Autodesk Inventor part; units mm, degrees
ref_plane "Work Plane1" through (0, 0, 12.7) normal (0, 0, 1) x (1, 0, 0)
ref_plane "Work Plane2" through (0, 0, -12.7) normal (0, 0, -1) x (-1, 0, 0)
ref_plane "YZ Plane" through (0, 0, 0) normal (1, 0, 0) x (0, 1, 0)
sketch "Sketch1" plane through (0, 0, 0) normal (0, 0, 1) x (1, 0, 0)
  line L0 (0, 0) -> (0, 12.7)
  line L1 (0, 12.7) -> (-25.952, 3.0759)
  line L2 (0, 0) -> (-25.4, 0)
  arc A0 (-25.952, 3.0759) -> (-25.4, 0) centre (-25.4, 1.5875) ccw
  dimension "d0" = 25.4
  dimension "d1" = 3.175
  dimension "d2" = 12.7
extrude "Extrusion1" add sketch "Sketch1" along normal mid plane 5.08
ref_plane "Work Plane1" through (0, 0, 12.7) normal (0, 0, 1) x (1, 0, 0)
sketch "Sketch2" plane through (0, 0, 12.7) normal (0, 0, 1) x (1, 0, 0)
  arc A0 (-32.2031, 3.109) -> (-31.75, 0) centre (-31.75, 1.5875) ccw
  line L0 (0, 0) -> (-31.75, 0)
  line L1 (0, 0) -> (0, 12.7)
  line L2 (0, 12.7) -> (-32.2031, 3.109)
  line L3 (0, 12.7) -> (-25.952, 3.0759) construction
  dimension "d6" = 3.175
  dimension "d7" = 31.75
ref_plane "Work Plane2" through (0, 0, -12.7) normal (0, 0, -1) x (-1, 0, 0)
sketch "Sketch3" plane through (0, 0, -12.7) normal (0, 0, -1) x (-1, 0, 0)
  line L0 (0, 12.7) -> (32.2031, 3.109)
  arc A0 (31.75, 0) -> (32.2031, 3.109) centre (31.75, 1.5875) ccw
  line L1 (0, 0) -> (31.75, 0)
  line L2 (0, 0) -> (0, 12.7)
loft "Loft1" add profiles "Sketch2" section 1 edges at (0, 6.35, 2.54) (-12.976, 7.888, 2.54) (-26.9625, 1.3071, 2.54) (-12.7, 0, 2.54)
loft "Loft2" add profiles "Sketch3" section 1 edges at (0, 6.35, -2.54) (-12.7, 0, -2.54) (-26.9625, 1.3071, -2.54) (-12.976, 7.888, -2.54)
sketch "Sketch4" plane through (0, 0, 12.7) normal (1, 0, 0) x (0, 0, -1)
  line L0 (15.24, 12.7) -> (10.16, 12.7) construction
  line L1 (10.16, 12.7) -> (0, 12.7) construction
  line L2 (0, 12.7) -> (0, 0) construction
  line L3 (0, 0) -> (25.4, 0) construction
  line L4 (25.4, 0) -> (25.4, 12.7) construction
  line L5 (15.24, 12.7) -> (25.4, 12.7) construction
  line L6 (0, 12.7) -> (12.7, 0) construction
  line L7 (12.7, 0) -> (25.4, 12.7) construction
  circle A0 centre (6.35, 6.35) radius 1.5875
  circle A1 centre (19.05, 6.35) radius 1.5875
  dimension "d17" = 3.175
  dimension "d18" = 3.175
extrude "Extrusion2" add sketch "Sketch4" along normal blind 6.35
properties part number "Bottom Pivot Mk1"
For this review, take the finished solid that the model builds, in its own axes (mm). A direction names the side the tool comes from. Round coordinates to 2 decimals unless told otherwise and drop trailing zeros. Loops run counter-clockwise (first coordinate to the right, second up) from the corner with the lowest first, then second, coordinate; pieces in that order, holes last.
Q1. Mouldability with a two-part tool opening along Z and no side actions: class faces 1 (the face through (-12, 4, 12.7)), 2 (the face through (-12, 0, 0)), 3 (the face through (3.131, 7.316, -5.09)) as +Z half, -Z half, draft (parallel to the pull), parting line (faces both ways), or undercut.
Result sheet:
face 1: +Z half
face 2: draft
face 3: undercut
Q2. Machinability: for faces 4 (the face through (3.13, 7.76, 5.62)), 5 (the face through (6.35, 6, -6)), 6 (the face through (-13, 5, -12.7)), 7 (the face through (-26.957, 1.277, -0.036)), 8 (the face through (-12.794, 7.955, -0.036)), which of the approach directions +Z, -Z, +X, -X, +Y, -Y give a long, thin tool a straight path to every point of the face, cutting with its end or side? Answer none if there is none.
Result sheet:
face 4: +X
face 5: +Z, -Z, +X, +Y, -Y
face 6: -Z, +X, -X, +Y, -Y
face 7: -X
face 8: -X, +Y
Q3. Add section A-A on z = -1.75. Write out the cut boundary in (x, y), plus the area to 3 significant figures.
Result sheet:
outline: (-25.95, 3.08) arc R1.59 ccw to (-25.4, 0) - (0, 0) - (0, 12.7) - close
area: 207 mm2
Q4. To check wall thickness, follow line 1 along Z through (x, y) = (3, 6.5); line 2 along Z through (x, y) = (-28, 1); line 3 along Y through (x, z) = (-25.5, -8). State the ranges of each line that lie inside material, in increasing order.
Result sheet:
line 1: z = -7.93 to -4.77, 4.77 to 7.93
line 2: z = -12.7 to -4.34, 4.34 to 12.7
line 3: y = 0 to 4.34
Q5. Insertion check: pin 1 Ø6 at (y, z) = (9.5, 0) entering from +X; pin 2 Ø2 at (x, z) = (-10, -9.5) entering from +Y; pin 3 Ø5 at (x, z) = (-9.5, 5) entering from +Y. Each pin has a flat end and moves straight along its axis. Give the tip position at first contact, or say it passes through.
Result sheet:
pin 1: stops at x = 0
pin 2: stops at y = 9.85
pin 3: stops at y = 10.26
